Part model, mm, in its own coordinate system. Face numbers are marked on the shaded views. A direction names the side the tool comes from. Round coordinates to 2 decimals unless told otherwise and drop trailing zeros. Write each loop counter-clockwise with the first axis right and the second up, starting at its lowest first coordinate (ties: lowest second). Pieces come first, ordered by that corner, then holes. Notation, with made-up numbers: M 55.5,-10 L 99.5,-10 A22 ccw 99.5,19 Z; hole C 15,19 d6. An arc over 180 degrees is marked long. One line per question, with ' | ' between items. Start each with the question number.
1) Saw through at D-D (z = 48). List the corners of the cut face in (x, y).
2) Mould opens along Z. For the marked faces 3, 4 and 5 say: pulls with the +Z half, pulls with the -Z half, needs draft (parallel to the pull), parting line crosses it, or undercut.
3) Drop flat-ended pins along their axis: pin 1 Ø7.5 at (x, y) = (-5.5, -4.5) entering from -Z; pin 2 Ø4 at (y, z) = (-3.5, 19) entering from +X; pin 3 Ø8 at (y, z) = (4.5, 58.5) entering from -X. Give the stop position or say it passes through.
4) Wall check: probe 1 along Y at (x, z) = (0, 50.8) (3 decimals); probe 2 along Z at (x, y) = (-2.25, 11); probe 3 along Y at (x, z) = (-9.2, 51.6) (3 decimals). Give the ranges that are in metal, low to high. Write a range as [from, to].
5) Tool access for the marked faces 1 and 2: list every direction of +Z, -Z, +X, -X, +Y, -Y with a clear straight run to the whole face (end or side of a thin tool).
6) Saw through at B-B (y = -4.75). List the corners of the cut face in (x, z), plus the area to 3 significant figures.
```python
from build123d import *

# Parameters (mm, degrees)
SKETCH1_R           = 12.5
BOSS_EXTRUDE1_DEPTH = 54.4
SKETCH2_R           = 3.45
BOSS_EXTRUDE2_DEPTH = 2.4
SKETCH3_R           = 2
BOSS_EXTRUDE3_DEPTH = 9.5
SKETCH4_W           = 6.273306019
SKETCH4_H           = 2.779797978
CUT_EXTRUDE1_DEPTH  = 9.5
SKETCH5_R           = 2.325
CUT_EXTRUDE2_DEPTH  = 4.45
SKETCH6_R           = 1.225
CUT_EXTRUDE3_DEPTH  = 4.45
SKETCH8_R           = 1
BOSS_EXTRUDE5_DEPTH = 7.7
SKETCH9_R           = 6.75
BOSS_EXTRUDE6_DEPTH = 6.7
SKETCH10_R          = 6.75
CUT_EXTRUDE5_DEPTH  = 2.2
SKETCH11_R          = 1
BOSS_EXTRUDE7_DEPTH = 2.2


with BuildPart() as part:
    # Sketch1 → Boss-Extrude1 (new body)
    with BuildSketch(Plane.XY):
        Circle(SKETCH1_R)
    extrude(amount=BOSS_EXTRUDE1_DEPTH)

    # Sketch2 → Boss-Extrude2 (add)
    with BuildSketch(Plane.XY.offset(54.4)):
        Circle(SKETCH2_R)
    extrude(amount=BOSS_EXTRUDE2_DEPTH)

    # Sketch3 → Boss-Extrude3 (add)
    with BuildSketch(Plane.XY.offset(56.8)):
        Circle(SKETCH3_R)
    extrude(amount=BOSS_EXTRUDE3_DEPTH)

    # Sketch4 → Cut-Extrude1 (cut)
    with BuildSketch(Plane.XY.offset(66.3)):
        with Locations((-0.006157841, 2.839898989)):
            Rectangle(SKETCH4_W, SKETCH4_H)
    extrude(amount=-CUT_EXTRUDE1_DEPTH, mode=Mode.SUBTRACT)

    # Sketch5 → Cut-Extrude2 (cut)
    with BuildSketch(Plane.XY.offset(54.4)):
        with Locations((0, 9.5)):
            Circle(SKETCH5_R)
        with Locations((0, -9.5)):
            Circle(SKETCH5_R)
    extrude(amount=-CUT_EXTRUDE2_DEPTH, mode=Mode.SUBTRACT)

    # Sketch6 → Cut-Extrude3 (cut)
    with BuildSketch(Plane.XY.offset(54.4)):
        with Locations((9.2, 0)):
            Circle(SKETCH6_R)
        with Locations((-9.2, 0)):
            Circle(SKETCH6_R)
    extrude(amount=-CUT_EXTRUDE3_DEPTH, mode=Mode.SUBTRACT)

    # Sketch8 → Boss-Extrude5 (add)
    with BuildSketch(Plane(origin=(0, 0, 0), x_dir=(-1, 0, 0), z_dir=(0, 0, -1))):
        with Locations(Location((0, 0, 0), (0, 0, 180))):
            Circle(SKETCH8_R)
    extrude(amount=BOSS_EXTRUDE5_DEPTH)

    # Sketch9 → Boss-Extrude6 (add)
    with BuildSketch(Plane(origin=(0, 0, 0), x_dir=(-1, 0, 0), z_dir=(0, 0, -1))):
        with Locations(Location((0, 0, 0), (0, 0, 180))):
            Circle(SKETCH9_R)
    extrude(amount=BOSS_EXTRUDE6_DEPTH)

    # Sketch10 → Cut-Extrude5 (cut)
    with BuildSketch(Plane(origin=(0, 0, 0), x_dir=(-1, 0, 0), z_dir=(0, 0, -1))):
        Circle(SKETCH10_R)
    extrude(amount=CUT_EXTRUDE5_DEPTH, mode=Mode.SUBTRACT)


with BuildPart() as cut_extrude5_piece_1:
    # of the separate pieces the step leaves, piece 1, a body of its own (cut_extrude5_pieces)
    add(part.part.solids().sort_by_distance((12.5, 0, 0))[0])



with BuildPart() as cut_extrude5_piece_2:
    # of the separate pieces the step leaves, piece 2, a body of its own (cut_extrude5_pieces)
    add(part.part.solids().sort_by_distance((6.75, 0, -2.2))[0])


with BuildPart() as cut_extrude5_piece_1_1:
    add(cut_extrude5_piece_1.part)

    add(cut_extrude5_piece_2.part)  # Boss-Extrude7 merges Cut-Extrude5 piece 2
    # Sketch11 → Boss-Extrude7 (add)
    with BuildSketch(Plane(origin=(0, 0, 0), x_dir=(-1, 0, 0), z_dir=(0, 0, -1))):
        with Locations(Location((0, 0, 0), (0, 0, 180))):
            Circle(SKETCH11_R)
    extrude(amount=BOSS_EXTRUDE7_DEPTH)


solid = cut_extrude5_piece_1_1.part
```
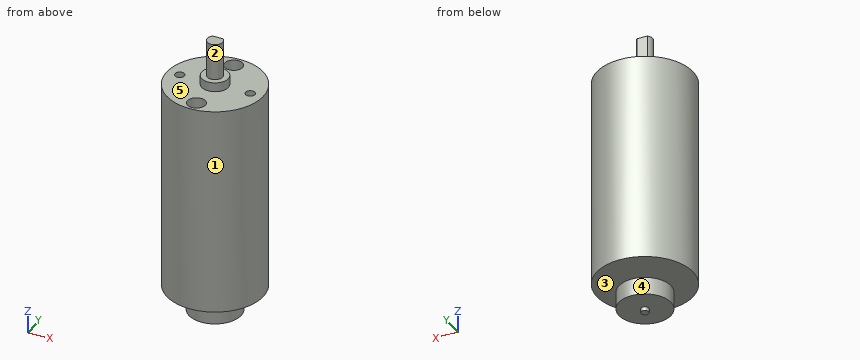
Answer key:
1) outline: C 0,0 d25
2) face 3: undercut | face 4: needs draft | face 5: pulls with the +Z half
3) pin 1: stops at z = -6.7 | pin 2: stops at x = 12.41 | pin 3: stops at x = -3.34
4) probe 1: y = [-12.5, -11.825], [-7.175, 7.175], [11.825, 12.5] | probe 2: z = [0, 54.4] | probe 3: y = [-8.462, -1.225], [1.225, 8.462]
5) face 1: +Z, -Z | face 2: +Z
6) outline: M -11.56,0 L 11.56,0 L 11.56,54.4 L -11.56,54.4 Z; M -4.8,-6.7 L 4.8,-6.7 L 4.8,-2.2 L -4.8,-2.2 Z | area: 1,300 mm2
